Can you work these out from the model? Positions are in its coordinate system, mm. Face numbers are marked on the shaded views. A direction names the side the tool comes from. Round coordinates to 2 decimals unless told otherwise and drop trailing zeros. Write each loop counter-clockwise with the first axis right and the second up, starting at its lowest first coordinate (ties: lowest second). Pieces come first, ordered by that corner, then holes. Notation, with made-up numbers: (76.5, 15.25) - (109.5, 15.25) arc R27 ccw to (109.5, 45.25) - close; hole circle Ø7 at (-34.75, 5.5). An arc over 180 degrees is marked (long way). One line per item, written item: value. Start each with the question number.
(1) On a 3-axis mill with a long thin cutter (end or side, diameter ignored), from which of +Z, -Z, +X, -X, +Y, -Y can I reach the whole of each face in a straight line? I mean the marked faces 1 and 2. Say none if no direction works.
(2) I want a section at B-B on x = 7.25. List the corners of the cut face in (y, z) for me (3 decimals), plus the area to 3 significant figures.
(3) I want a section at A-A on y = 3.5. List the corners of the cut face in (x, z) for me (3 decimals), plus the area to 3 significant figures.
(4) If I drill on L1, parallel to Z at x = 7.5, y = 2.5 (3 decimals); L2, parallel to X at y = 3, z = -4.5 (3 decimals); L3, parallel to Y at x = 1.25, z = -4.25, over which ranges is the centre line in solid material (lowest first)? Write a range as from..to.
(5) I'm going to push a flat-ended pin straight in: pin 1 Ø3 at (x, z) = (8.5, 2.5) entering from +Y. Where does the tip first touch, or does it pass through?
(6) Thinking about a two-plate mould opening in Z: for the marked faces 3, 4, 5 and 6, which applies, +Z half, -Z half, draft (parallel to the pull), parting line (faces both ways), or undercut?
(7) I want a section at C-C on y = 10.5. List the corners of the cut face in (x, z) for me (3 decimals).
(8) I want a section at D-D on z = 5. List the corners of the cut face in (x, y) for me (3 decimals), plus the area to 3 significant figures.
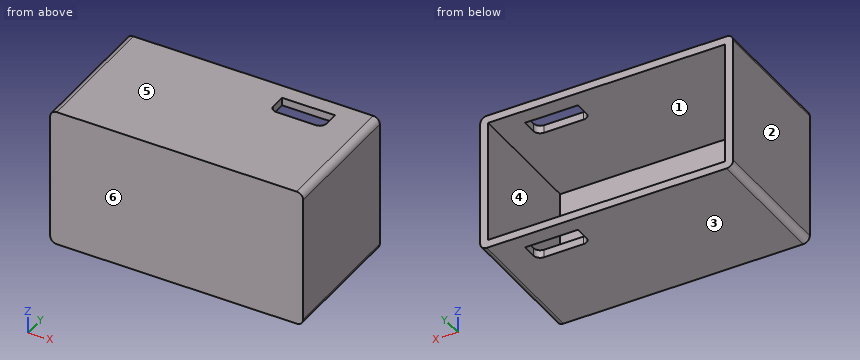
from build123d import *

# Parameters (mm, degrees)
SKETCH1_W           = 24.2700048
SKETCH1_H           = 13.3700012
BOSS_EXTRUDE1_DEPTH = 12.7
SHELL1_T            = -0.762
FILLET1_R           = 0.635
SKETCH2_W           = 5.08
SKETCH2_H           = 2.032
CUT_EXTRUDE1_DEPTH  = 23.074990721
FILLET2_R           = 0.635


with BuildPart() as part:
    # Sketch1 → Boss-Extrude1 (new body)
    with BuildSketch(Plane(origin=(0, 0, 0), x_dir=(1, 0, 0), z_dir=(0, 1, 0))):
        Rectangle(SKETCH1_W, SKETCH1_H)
    extrude(amount=BOSS_EXTRUDE1_DEPTH)

    # Shell1
    shell1_openings = [part.faces().sort_by_distance(p)[0] for p in [
        (0, 12.7, 0),
    ]]
    offset(amount=SHELL1_T, openings=shell1_openings, kind=Kind.INTERSECTION)

    # Fillet1
    fillet1_edges = [part.edges().sort_by_distance(p)[0] for p in [
        (12.1350024, 6.35, 6.6850006),
        (-12.1350024, 6.35, 6.6850006),
        (-12.1350024, 6.35, -6.6850006),
        (12.1350024, 6.35, -6.6850006),
    ]]
    fillet(fillet1_edges, radius=FILLET1_R)

    # Sketch2 → Cut-Extrude1 (cut, through all)
    with BuildSketch(Plane.XY.offset(6.6850006)):
        with Locations((6.1660024, 10.16)):
            Rectangle(SKETCH2_W, SKETCH2_H)
    extrude(amount=-CUT_EXTRUDE1_DEPTH, mode=Mode.SUBTRACT)

    # Fillet2
    fillet2_edges = [part.edges().sort_by_distance(p)[0] for p in [
        (8.7060024, 9.144, -6.3040006),
        (3.6260024, 9.144, -6.3040006),
        (8.7060024, 9.144, 6.3040006),
        (3.6260024, 9.144, 6.3040006),
    ]]
    fillet(fillet2_edges, radius=FILLET2_R)


solid = part.part
Established:
1. face 1: +Y
1. face 2: +Z, -Z, -X, +Y, -Y
2. outline: (0, -6.685) - (9.144, -6.685) - (9.144, -5.923) - (0.762, -5.923) - (0.762, 5.923) - (9.144, 5.923) - (9.144, 6.685) - (0, 6.685) - close; (11.176, -6.685) - (12.7, -6.685) - (12.7, -5.923) - (11.176, -5.923) - close; (11.176, 5.923) - (12.7, 5.923) - (12.7, 6.685) - (11.176, 6.685) - close
2. area: 25.3 mm2
3. outline: (-12.135, -6.05) arc R0.635 ccw to (-11.5, -6.685) - (11.5, -6.685) arc R0.635 ccw to (12.135, -6.05) - (12.135, 6.05) arc R0.635 ccw to (11.5, 6.685) - (-11.5, 6.685) arc R0.635 ccw to (-12.135, 6.05) - close; hole (-11.373, -5.923) - (11.373, -5.923) - (11.373, 5.923) - (-11.373, 5.923) - close
3. area: 54.7 mm2
4. L1: -6.685..-5.923, 5.923..6.685
4. L2: -12.135..-11.373, 11.373..12.135
4. L3: 0..0.76
5. pin 1: y = 0.76
6. face 3: -Z half
6. face 4: undercut
6. face 5: +Z half
6. face 6: draft
7. outline: (-12.135, -6.05) arc R0.635 ccw to (-11.5, -6.685) - (3.626, -6.685) - (3.626, -5.923) - (-11.373, -5.923) - (-11.373, 5.923) - (3.626, 5.923) - (3.626, 6.685) - (-11.5, 6.685) arc R0.635 ccw to (-12.135, 6.05) - close; (8.706, -6.685) - (11.5, -6.685) arc R0.635 ccw to (12.135, -6.05) - (12.135, 6.05) arc R0.635 ccw to (11.5, 6.685) - (8.706, 6.685) - (8.706, 5.923) - (11.373, 5.923) - (11.373, -5.923) - (8.706, -5.923) - close
8. outline: (-12.135, 0) - (12.135, 0) - (12.135, 12.7) - (11.373, 12.7) - (11.373, 0.762) - (-11.373, 0.762) - (-11.373, 12.7) - (-12.135, 12.7) - close
8. area: 36.7 mm2
